from build123d import *

# Parameters (mm, degrees)
SKETCH_1_R      = 1.6
SKETCH_1_R_2    = 1.5
EXTRUDE_1_DEPTH = 5
FILLET_1_R      = 5


with BuildPart() as part:
    # ｽｹｯﾁ1 → ﾎﾞｽ - 押し出し1 (new body)
    with BuildSketch(Plane(origin=(0, 0, 0), x_dir=(1, 0, 0), z_dir=(0, 1, 0))):
        with BuildLine():
            Line((-13.75, -32.5), (-13.75, -42.5))
            Line((-13.75, -42.5), (13.75, -42.5))
            Line((13.75, -42.5), (13.75, 42.5))
            ThreePointArc((13.75, 42.5), (6.25, 50), (-1.25, 42.5))
            Line((-1.25, 42.5), (-1.351786435, 42.5))
            Line((-1.351786435, 42.5), (-13.75, -32.5))
        make_face()
        with Locations(Location((-8.75, -37.5, 0), (0, 0, 270))):
            Circle(SKETCH_1_R, mode=Mode.SUBTRACT)
        with Locations(Location((8.75, -37.5, 0), (0, 0, 270))):
            Circle(SKETCH_1_R, mode=Mode.SUBTRACT)
        with Locations(Location((8.75, -17.5, 0), (0, 0, 270))):
            Circle(SKETCH_1_R_2, mode=Mode.SUBTRACT)
        with Locations(Location((8.75, -2.5, 0), (0, 0, 270))):
            Circle(SKETCH_1_R_2, mode=Mode.SUBTRACT)
    extrude(amount=EXTRUDE_1_DEPTH)

    # ﾌｨﾚｯﾄ1
    fillet_1_edges = [part.edges().sort_by_distance(p)[0] for p in [
        (13.75, 2.5, 42.5),
        (-13.75, 2.5, 42.5),
    ]]
    fillet(fillet_1_edges, radius=FILLET_1_R)


solid = part.part
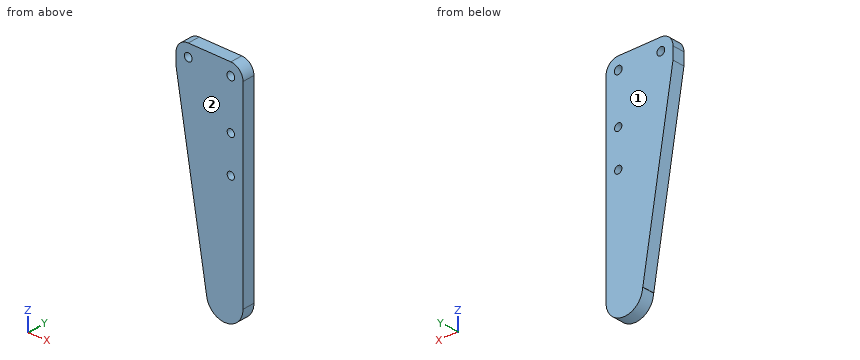
Build history of the part. All positions in model axes, mm. Face numbers are marked on the shaded views. Coordinates: 2 decimals unless noted, no trailing zeros. Write each loop counter-clockwise with the first axis right and the second up, starting at its lowest first coordinate (ties: lowest second). Pieces come first, ordered by that corner, then holes.
(1) Drill centre lines: line 1 (X direction, y = 2.05, z = 37.5); line 2 (X direction, y = 0.35, z = 18); line 3 (Z direction, x = 0.5, y = 1.55). Where is each one in solid material? Low to high.
(2) Cut at C-C on z = 17.5. List the corners of the cut face in (x, y).
(3) Mould opens along Y. For the marked faces 1 and 2 say: pulls with the +Y half, pulls with the -Y half, needs draft (parallel to the pull), parting line crosses it, or undercut.
(4) Cut at A-A on y = 3.6. List the corners of the cut face in (x, z).
(5) Cut at D-D on x = -0.25. List the corners of the cut face in (y, z), and give its area (3 significant figures).
(6) Cut at B-B on z = 2.5. List the corners of the cut face in (x, y), and give its area (3 significant figures).
(7) Pin check, flat tips, straight feed: pin 1 Ø2.5 at (x, z) = (8.75, 2.5) entering from -Y; pin 2 Ø2 at (y, z) = (3.5, 9) entering from -X. Stop position of each tip, or through.
Working result:
1. line 1: x = -13.75 to -10.35, -7.15 to 7.15, 10.35 to 13.75
1. line 2: x = -11.35 to 7.34, 10.16 to 13.75
1. line 3: z = -47.32 to 42.5
2. outline: (-11.27, 0) - (7.25, 0) - (7.25, 5) - (-11.27, 5) - close; (10.25, 0) - (13.75, 0) - (13.75, 5) - (10.25, 5) - close
3. face 1: pulls with the +Y half
3. face 2: pulls with the -Y half
4. outline: (-13.75, 32.5) - (-1.35, -42.5) - (-1.25, -42.5) arc R7.5 ccw to (13.75, -42.5) - (13.75, 37.5) arc R5 ccw to (8.75, 42.5) - (-8.75, 42.5) arc R5 ccw to (-13.75, 37.5) - close; hole circle Ø3.2 at (-8.75, 37.5); hole circle Ø3.2 at (8.75, 37.5); hole circle Ø3 at (8.75, 2.5); hole circle Ø3 at (8.75, 17.5)
5. outline: (0, -46.24) - (5, -46.24) - (5, 42.5) - (0, 42.5) - close
5. area: 444 mm2
6. outline: (-8.79, 0) - (7.25, 0) - (7.25, 5) - (-8.79, 5) - close; (10.25, 0) - (13.75, 0) - (13.75, 5) - (10.25, 5) - close
6. area: 97.7 mm2
7. pin 1: passes through
7. pin 2: stops at x = -10.03
